Input: part model. Units: mm. Frame: model coordinates. Coordinates: 2 decimals unless noted, no trailing zeros. Loops run counter-clockwise (first coordinate to the right, second up) from the corner with the lowest first, then second, coordinate; pieces in that order, holes last. Notation, with made-up numbers: (6, 5) -> (10, 5) arc R20 ccw to (10, 14) -> close; hole circle Ø11 at (-10.75, 36.5). An arc over 180 degrees is marked (long way). Answer as a JSON object with one key per item and string values.
from build123d import *

# Parameters (mm, degrees)
F0_W     = 360
F0_H     = 220
F0_R     = 3.5
F0_W_2   = 20
F0_H_2   = 100
F1_DEPTH = 8


with BuildPart() as f1:
    # F0 (on Top) → F1 (new body)
    with BuildSketch(Plane.XY):
        Rectangle(F0_W, F0_H)
        with Locations((-135, -90)):
            Circle(F0_R, mode=Mode.SUBTRACT)
        with Locations((-105, -90)):
            Circle(F0_R, mode=Mode.SUBTRACT)
        with Locations((-135, -60)):
            Circle(F0_R, mode=Mode.SUBTRACT)
        with Locations((-105, -60)):
            Circle(F0_R, mode=Mode.SUBTRACT)
        with Locations((-75, -90)):
            Circle(F0_R, mode=Mode.SUBTRACT)
        with Locations((-45, -90)):
            Circle(F0_R, mode=Mode.SUBTRACT)
        with Locations((-15, -90)):
            Circle(F0_R, mode=Mode.SUBTRACT)
        with Locations((-75, -60)):
            Circle(F0_R, mode=Mode.SUBTRACT)
        with Locations((-45, -60)):
            Circle(F0_R, mode=Mode.SUBTRACT)
        with Locations((-15, -60)):
            Circle(F0_R, mode=Mode.SUBTRACT)
        with Locations((-135, -30)):
            Circle(F0_R, mode=Mode.SUBTRACT)
        with Locations((-105, -30)):
            Circle(F0_R, mode=Mode.SUBTRACT)
        with Locations((-75, -30)):
            Circle(F0_R, mode=Mode.SUBTRACT)
        with Locations((-45, -30)):
            Circle(F0_R, mode=Mode.SUBTRACT)
        with Locations((-15, -30)):
            Circle(F0_R, mode=Mode.SUBTRACT)
        with Locations((15, -90)):
            Circle(F0_R, mode=Mode.SUBTRACT)
        with Locations((45, -90)):
            Circle(F0_R, mode=Mode.SUBTRACT)
        with Locations((75, -90)):
            Circle(F0_R, mode=Mode.SUBTRACT)
        with Locations((15, -60)):
            Circle(F0_R, mode=Mode.SUBTRACT)
        with Locations((45, -60)):
            Circle(F0_R, mode=Mode.SUBTRACT)
        with Locations((75, -60)):
            Circle(F0_R, mode=Mode.SUBTRACT)
        with Locations((105, -90)):
            Circle(F0_R, mode=Mode.SUBTRACT)
        with Locations((135, -90)):
            Circle(F0_R, mode=Mode.SUBTRACT)
        with Locations((105, -60)):
            Circle(F0_R, mode=Mode.SUBTRACT)
        with Locations((135, -60)):
            Circle(F0_R, mode=Mode.SUBTRACT)
        with Locations((15, -30)):
            Circle(F0_R, mode=Mode.SUBTRACT)
        with Locations((45, -30)):
            Circle(F0_R, mode=Mode.SUBTRACT)
        with Locations((75, -30)):
            Circle(F0_R, mode=Mode.SUBTRACT)
        with Locations((105, -30)):
            Circle(F0_R, mode=Mode.SUBTRACT)
        with Locations((135, -30)):
            Circle(F0_R, mode=Mode.SUBTRACT)
        with Locations((-160, 0)):
            Rectangle(F0_W_2, F0_H_2, mode=Mode.SUBTRACT)
        with Locations((-135, 0)):
            Circle(F0_R, mode=Mode.SUBTRACT)
        with Locations((-105, 0)):
            Circle(F0_R, mode=Mode.SUBTRACT)
        with Locations((-135, 30)):
            Circle(F0_R, mode=Mode.SUBTRACT)
        with Locations((-105, 30)):
            Circle(F0_R, mode=Mode.SUBTRACT)
        with Locations((-75, 0)):
            Circle(F0_R, mode=Mode.SUBTRACT)
        with Locations((-45, 0)):
            Circle(F0_R, mode=Mode.SUBTRACT)
        with Locations((-15, 0)):
            Circle(F0_R, mode=Mode.SUBTRACT)
        with Locations((-75, 30)):
            Circle(F0_R, mode=Mode.SUBTRACT)
        with Locations((-45, 30)):
            Circle(F0_R, mode=Mode.SUBTRACT)
        with Locations((-15, 30)):
            Circle(F0_R, mode=Mode.SUBTRACT)
        with Locations((-135, 60)):
            Circle(F0_R, mode=Mode.SUBTRACT)
        with Locations((-105, 60)):
            Circle(F0_R, mode=Mode.SUBTRACT)
        with Locations((-135, 90)):
            Circle(F0_R, mode=Mode.SUBTRACT)
        with Locations((-105, 90)):
            Circle(F0_R, mode=Mode.SUBTRACT)
        with Locations((-75, 60)):
            Circle(F0_R, mode=Mode.SUBTRACT)
        with Locations((-45, 60)):
            Circle(F0_R, mode=Mode.SUBTRACT)
        with Locations((-15, 60)):
            Circle(F0_R, mode=Mode.SUBTRACT)
        with Locations((-75, 90)):
            Circle(F0_R, mode=Mode.SUBTRACT)
        with Locations((-45, 90)):
            Circle(F0_R, mode=Mode.SUBTRACT)
        with Locations((-15, 90)):
            Circle(F0_R, mode=Mode.SUBTRACT)
        with Locations((15, 0)):
            Circle(F0_R, mode=Mode.SUBTRACT)
        with Locations((45, 0)):
            Circle(F0_R, mode=Mode.SUBTRACT)
        with Locations((75, 0)):
            Circle(F0_R, mode=Mode.SUBTRACT)
        with Locations((15, 30)):
            Circle(F0_R, mode=Mode.SUBTRACT)
        with Locations((45, 30)):
            Circle(F0_R, mode=Mode.SUBTRACT)
        with Locations((75, 30)):
            Circle(F0_R, mode=Mode.SUBTRACT)
        with Locations((105, 0)):
            Circle(F0_R, mode=Mode.SUBTRACT)
        with Locations((135, 0)):
            Circle(F0_R, mode=Mode.SUBTRACT)
        with Locations((160, 0)):
            Rectangle(F0_W_2, F0_H_2, mode=Mode.SUBTRACT)
        with Locations((105, 30)):
            Circle(F0_R, mode=Mode.SUBTRACT)
        with Locations((135, 30)):
            Circle(F0_R, mode=Mode.SUBTRACT)
        with Locations((15, 60)):
            Circle(F0_R, mode=Mode.SUBTRACT)
        with Locations((45, 60)):
            Circle(F0_R, mode=Mode.SUBTRACT)
        with Locations((75, 60)):
            Circle(F0_R, mode=Mode.SUBTRACT)
        with Locations((15, 90)):
            Circle(F0_R, mode=Mode.SUBTRACT)
        with Locations((45, 90)):
            Circle(F0_R, mode=Mode.SUBTRACT)
        with Locations((75, 90)):
            Circle(F0_R, mode=Mode.SUBTRACT)
        with Locations((105, 60)):
            Circle(F0_R, mode=Mode.SUBTRACT)
        with Locations((135, 60)):
            Circle(F0_R, mode=Mode.SUBTRACT)
        with Locations((105, 90)):
            Circle(F0_R, mode=Mode.SUBTRACT)
        with Locations((135, 90)):
            Circle(F0_R, mode=Mode.SUBTRACT)
    extrude(amount=F1_DEPTH)


solid = f1.part
1. Line query: line 1 along X through (y, z) = (-42.5, 1.25). Output: solid intervals per line, ascending.
Reply:
{"line 1": "x = -180 to -170, -150 to 150, 170 to 180"}
2. Mould query, pull axis X, two halves, no side actions, for faces 1 (the face through (42.42, 32.365, 3.944)), 2 (the face through (-3, 2, 8)). Classes: pulls with the +X half, pulls with the -X half, needs draft (parallel to the pull), parting line crosses it, or undercut.
Reply:
{"face 1": "undercut", "face 2": "needs draft"}
3. Section query A-A (x = 75). Count the separate pieces of the cut face and the enclosed holes in it, plus the area to 3 significant figures.
Reply:
{"separate pieces": "8", "enclosed holes": "0", "area": "1,370 mm2"}
4. Section query B-B (y = 8.5). Return loops of the section in (x, z), plus the area to 3 significant figures.
Reply:
{"outline": "(-180, 0) -> (-170, 0) -> (-170, 8) -> (-180, 8) -> close; (-150, 0) -> (150, 0) -> (150, 8) -> (-150, 8) -> close; (170, 0) -> (180, 0) -> (180, 8) -> (170, 8) -> close", "area": "2,560 mm2"}
